```python
from build123d import *

# Parameters (mm, degrees)
SKETCH2_R           = 17
BOSS_EXTRUDE1_DEPTH = 25
SKETCH2_3_R         = 19
SKETCH2_3_R_2       = 17
BOSS_EXTRUDE2_DEPTH = 8
BOSS_EXTRUDE3_DEPTH = 15
SKETCH4_R           = 16
BOSS_EXTRUDE4_DEPTH = 15
SKETCH5_R           = 17
BOSS_EXTRUDE5_DEPTH = 5
BOSS_EXTRUDE6_DEPTH = 15
SKETCH7_R           = 16
BOSS_EXTRUDE7_DEPTH = 30
BOSS_EXTRUDE8_DEPTH = 15
SKETCH9_R           = 17
BOSS_EXTRUDE9_DEPTH = 2.5


with BuildPart() as part:
    # Sketch2 → Boss-Extrude1 (new body)
    with BuildSketch(Plane(origin=(0, 0, 0), x_dir=(0, 0, -1), z_dir=(1, 0, 0))):
        Circle(SKETCH2_R)
    extrude(amount=-BOSS_EXTRUDE1_DEPTH)

    # Sketch2_3 → Boss-Extrude2 (add)
    with BuildSketch(Plane(origin=(0, 0, 0), x_dir=(0, 0, -1), z_dir=(1, 0, 0))):
        Circle(SKETCH2_3_R)
        Circle(SKETCH2_3_R_2, mode=Mode.SUBTRACT)
        Circle(SKETCH2_3_R_2)
    extrude(amount=BOSS_EXTRUDE2_DEPTH)

    # Sketch3 → Boss-Extrude3 (add)
    with BuildSketch(Plane(origin=(8, 0, 0), x_dir=(0, 0, -1), z_dir=(1, 0, 0))):
        with BuildLine():
            ThreePointArc((13.668094758, 40.943123461), (0, 46), (-13.668094758, 40.943123461))
            ThreePointArc((-13.668094758, 40.943123461), (-33.683444249, 16.469257624), (-44, -13.416407865))
            ThreePointArc((-44, -13.416407865), (0, -46), (44, -13.416407865))
            ThreePointArc((44, -13.416407865), (33.683444249, 16.469257624), (13.668094758, 40.943123461))
        make_face()
    boss_extrude3 = extrude(amount=BOSS_EXTRUDE3_DEPTH)

    # Sketch4 → Boss-Extrude4 (add)
    with BuildSketch(Plane(origin=(23, 0, 0), x_dir=(0, 0, -1), z_dir=(1, 0, 0))):
        with Locations(Location((0, 25, 0), (0, 0, 180))):
            Circle(SKETCH4_R)
    boss_extrude4 = extrude(amount=BOSS_EXTRUDE4_DEPTH)

    # Mirror1: Boss-Extrude3, Boss-Extrude4 across plane
    add(boss_extrude3.mirror(Plane(origin=(38, 25, 0), x_dir=(0, 0, 1), z_dir=(1, 0, 0))))
    add(boss_extrude4.mirror(Plane(origin=(38, 25, 0), x_dir=(0, 0, 1), z_dir=(1, 0, 0))))

    # Sketch5 → Boss-Extrude5 (add)
    with BuildSketch(Plane(origin=(68, 0, 0), x_dir=(0, 0, -1), z_dir=(1, 0, 0))):
        Circle(SKETCH5_R)
    extrude(amount=BOSS_EXTRUDE5_DEPTH)

    # Sketch6 → Boss-Extrude6 (add)
    with BuildSketch(Plane(origin=(73, 0, 0), x_dir=(0, 0, -1), z_dir=(1, 0, 0))):
        with BuildLine():
            ThreePointArc((-13.668094758, -40.943123461), (0, -46), (13.668094758, -40.943123461))
            ThreePointArc((13.668094758, -40.943123461), (33.683444249, -16.469257624), (44, 13.416407865))
            ThreePointArc((44, 13.416407865), (0, 46), (-44, 13.416407865))
            ThreePointArc((-44, 13.416407865), (-33.683444249, -16.469257624), (-13.668094758, -40.943123461))
        make_face()
    extrude(amount=BOSS_EXTRUDE6_DEPTH)

    # Sketch7 → Boss-Extrude7 (add)
    with BuildSketch(Plane(origin=(88, 0, 0), x_dir=(0, 0, -1), z_dir=(1, 0, 0))):
        with Locations((0, -25)):
            Circle(SKETCH7_R)
    extrude(amount=BOSS_EXTRUDE7_DEPTH)

    # Sketch8 → Boss-Extrude8 (add)
    with BuildSketch(Plane(origin=(118, 0, 0), x_dir=(0, 0, -1), z_dir=(1, 0, 0))):
        with BuildLine():
            ThreePointArc((-13.668094758, -40.943123461), (0, -46), (13.668094758, -40.943123461))
            ThreePointArc((13.668094758, -40.943123461), (33.683444249, -16.469257624), (44, 13.416407865))
            ThreePointArc((44, 13.416407865), (0, 46), (-44, 13.416407865))
            ThreePointArc((-44, 13.416407865), (-33.683444249, -16.469257624), (-13.668094758, -40.943123461))
        make_face()
    extrude(amount=BOSS_EXTRUDE8_DEPTH)

    # Sketch9 → Boss-Extrude9 (add)
    with BuildSketch(Plane(origin=(133, 0, 0), x_dir=(0, 0, -1), z_dir=(1, 0, 0))):
        Circle(SKETCH9_R)
    extrude(amount=BOSS_EXTRUDE9_DEPTH)

    # Mirror2: part across plane


with BuildPart() as part_1:
    add(part.part)
    add(part.part.mirror(Plane(origin=(135.5, 0, 0), x_dir=(0, 0, 1), z_dir=(1, 0, 0))))


solid = part_1.part
```
Read the model definition and answer for the solid it produces. Units are mm, in the model's axes. A direction names the side the tool comes from. Give positions to 0.01 mm unless a question says otherwise; leave off trailing zeros. Order: outer loops, then holes, each group sorted by start corner. A loop starts at its lowest first (then second) coordinate and runs counter-clockwise, first axis right, second up. Notation, with made-up numbers: (27, 63) -> (45, 63) arc R28 ccw to (45, 81) -> close; hole circle Ø6 at (-27.5, -26). An arc over 180 degrees is marked (long way). One line per item, written item: value. Start each with the question number.
(1) For a pull along X with two mould halves and no side action, classify faces 1 (the flat face through (296, 0, 0)), 2 (the flat face through (203, -20, 1)), 3 (the cylindrical face through (255.605, -45.993, 0.821)) as released by +X, released by -X, zero draft, split by the parting line, or undercut.
(2) A tool of negligible diameter and unlimited length cuts with its end or side. For faces 4 (the cylindrical face through (146, -46, 0)), 5 (the cylindrical face through (145.605, -16.857, -33.466)), 6 (the cylindrical face through (200.535, 14.334, -9.139)), 7 (the cylindrical face through (267.056, -16.856, -8.767)), from which of +Z, -Z, +X, -X, +Y, -Y can it reach the whole face along a straight path? Write none if from no direction.
(3) The part is cut by section A-A (z = -30). State how many separate pieces and enclosed holes the cut face has, and give its area (3 significant figures).
(4) Flat-ended cylindrical pins translate along their axes: P1, Ø3, axis at y = 18.5, z = -15.5, coming from the +X side; P2, Ø1, axis at x = 94, z = 6.5, coming from the +Y side; P3, Ø5, axis at x = 129, y = 3.5, coming from the +Z side. Find the tip coordinate at first contact, or state that the pin passes through.
(5) Straight lines are drawn through the part: L1, parallel to X at y = 38.5, z = 1; L2, parallel to X at y = -23.5, z = 39.5; L3, parallel to X at y = 36, z = -25. For each, find the intervals that lie inside material, in ascending order.
(6) The part is cut by section D-D (x = 76). Determine the outline of the cut face in (y, z), and give its area (3 significant figures).
Taken from the geometry:
1. face 1: released by +X
1. face 2: undercut
1. face 3: zero draft
2. face 4: -Y
2. face 5: -Z, -Y
2. face 6: none
2. face 7: +X
3. separate pieces: 8
3. enclosed holes: 0
3. area: 6,880 mm^2
4. P1: x = 263
4. P2: y = -10.17
4. P3: z = 42.51
5. L1: 8 to 68, 73 to 88, 118 to 133, 138 to 153, 183 to 198, 203 to 263
5. L2: 8 to 23, 53 to 68, 203 to 218, 248 to 263
5. L3: 73 to 88, 118 to 133, 138 to 153, 183 to 198
6. outline: (-40.94, -13.67) arc R90 ccw to (13.42, -44) arc R46 ccw to (13.42, 44) arc R90 ccw to (-40.94, 13.67) arc R21 ccw to start
6. area: 5,800 mm^2
